Part print with two shaded views. Sizes in mm from the minimum x, y, z corner. Round coordinates to 2 decimals unless told otherwise and drop trailing zeros. Loops run counter-clockwise (first coordinate to the right, second up) from the corner with the lowest first, then second, coordinate; pieces in that order, holes last. Notation, with made-up numbers: (0.25, 75) -> (37.25, 75) arc R16 ccw to (37.25, 81) -> close; hole circle Ø9 at (89.5, -23.5). An arc over 180 degrees is marked (long way). Use a Markdown table: item, result. Add a question column.
Item 1: Flat gauge pin, fed straight in: pin 1 (1 mm diameter, centred on x = 7, z = 4, fed in from -Y). Where does the tip first touch, or does it go through?
Item 2: Cut at B-B, the plane z = 3. List the corners of the cut face in (x, y), plus the area to 3 significant figures.
Item 3: Cut at D-D, the plane x = 50. List the corners of the cut face in (y, z).
Item 4: Probe line 1 (Y direction, x = 30, z = 3.35); line 2 (X direction, y = 10.5, z = 2.9); line 3 (Y direction, x = 50, z = 3.35). List the from-to ranges inside material, lowest first. Write a range as [from, to].
Item 5: Cut at A-A, the plane x = 30. List the corners of the cut face in (y, z), plus the area to 3 significant figures.
Item 6: Cut at C-C, the plane y = 82.5. List the corners of the cut face in (x, z).
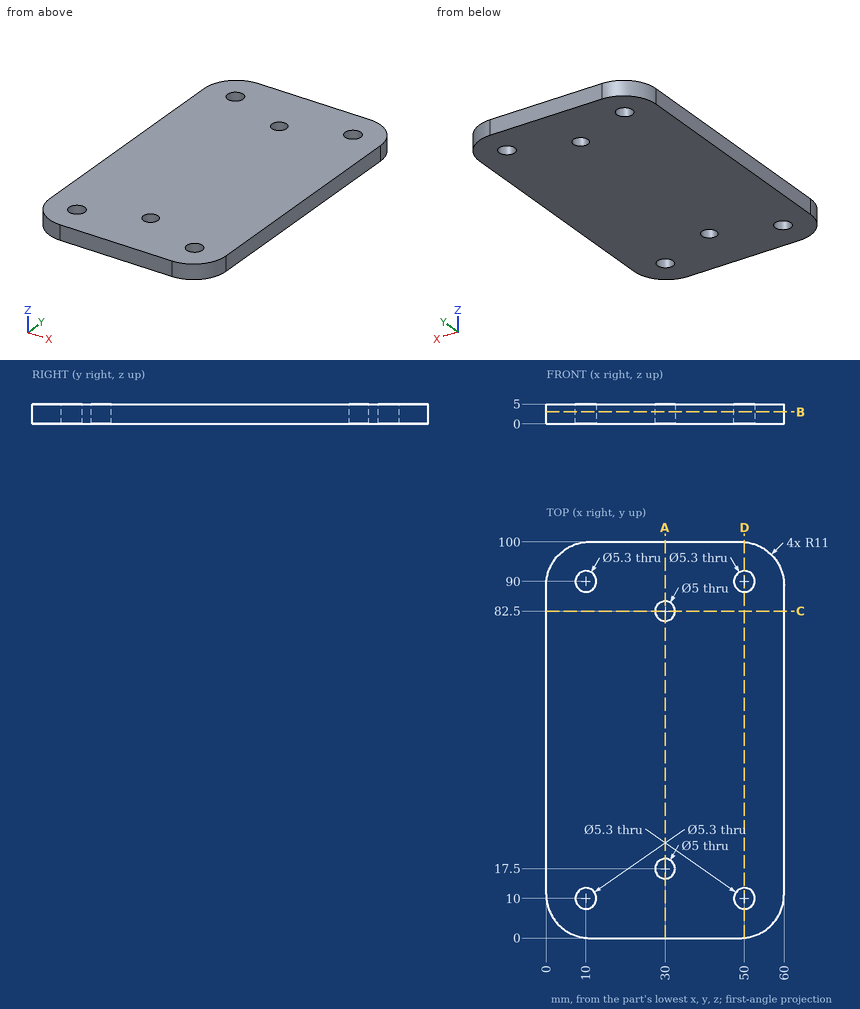
A:
| question | item | result |
|---|---|---|
| 1 | pin 1 | stops at y = 0.57 |
| 2 | outline | (0, 11) arc R11 ccw to (11, 0) -> (49, 0) arc R11 ccw to (60, 11) -> (60, 89) arc R11 ccw to (49, 100) -> (11, 100) arc R11 ccw to (0, 89) -> close; hole circle Ø5.3 at (10, 10); hole circle Ø5.3 at (10, 90); hole circle Ø5 at (30, 17.5); hole circle Ø5 at (30, 82.5); hole circle Ø5.3 at (50, 10); hole circle Ø5.3 at (50, 90) |
| 2 | area | 5,770 mm^2 |
| 3 | outline | (0.05, 0) -> (7.35, 0) -> (7.35, 5) -> (0.05, 5) -> close; (12.65, 0) -> (87.35, 0) -> (87.35, 5) -> (12.65, 5) -> close; (92.65, 0) -> (99.95, 0) -> (99.95, 5) -> (92.65, 5) -> close |
| 4 | line 1 | y = [0, 15], [20, 80], [85, 100] |
| 4 | line 2 | x = [0.01, 7.4], [12.6, 47.4], [52.6, 59.99] |
| 4 | line 3 | y = [0.05, 7.35], [12.65, 87.35], [92.65, 99.95] |
| 5 | outline | (0, 0) -> (15, 0) -> (15, 5) -> (0, 5) -> close; (20, 0) -> (80, 0) -> (80, 5) -> (20, 5) -> close; (85, 0) -> (100, 0) -> (100, 5) -> (85, 5) -> close |
| 5 | area | 450 mm^2 |
| 6 | outline | (0, 0) -> (27.5, 0) -> (27.5, 5) -> (0, 5) -> close; (32.5, 0) -> (60, 0) -> (60, 5) -> (32.5, 5) -> close |
